Autodesk Inventor part; units mm, degrees
ref_plane "YZ Plane" through (0, 0, 0) normal (1, 0, 0) x (0, 1, 0)
ref_plane "XZ Plane" through (0, 0, 0) normal (0, 1, 0) x (-1, 0, 0)
ref_plane "XY Plane" through (0, 0, 0) normal (0, 0, 1) x (1, 0, 0)
sketch "Sketch1" plane through (0, 0, 0) normal (0, 0, 1) x (1, 0, 0)
  arc A0 (-31, -3) -> (-3, -31) centre (-3, -3) ccw
  line L0 (-31, -3) -> (-31, 0)
  line L1 (-31, 0) -> (0, 0)
  line L2 (0, 0) -> (0, -31)
  line L3 (0, -31) -> (-3, -31)
  line L4 (-31, -3) -> (-3, -3)
  line L5 (-3, -3) -> (-3, -31)
  circle A1 centre (-14.34, -15.19) radius 5.05
  circle A2 centre (-14.34, -15.19) radius 1.25
  arc A3 (0, -30.38) -> (-28.68, 0) centre (-14.34, -15.19) ccw
  dimension "wallThickness" = 3
  dimension "d1" = 3
  dimension "width" = 31
  dimension "d3" = 31
  dimension "diameter" = 10.1
  dimension "d5" = 12.19
  dimension "d6" = 11.34
  dimension "centerHoleDia" = 2.5
  dimension "setScrewRingRad" = 20.8895
extrude "Extrusion1" add sketch "Sketch1" against normal blind 3 contours L4 L5 A0 | L0 L1 L2 L3 L5 L4 | A3 L1 | L2 A3 | A1 | A2
extrude "Extrusion2" add sketch "Sketch1" along normal blind 20 contours L0 L1 L2 L3 L5 L4 | A3 L1 | L2 A3
extrude "Extrusion3" add sketch "Sketch1" along normal blind 15 contours A1 | A2
extrude "Extrusion7" cut sketch "Sketch1" along normal through all both and the other way through all contours A2
equation "\"d1\" = wallThickness"
equation "\"d3\" = width"
equation "\"d7\" = wallThickness"
properties part number "tv-mount"
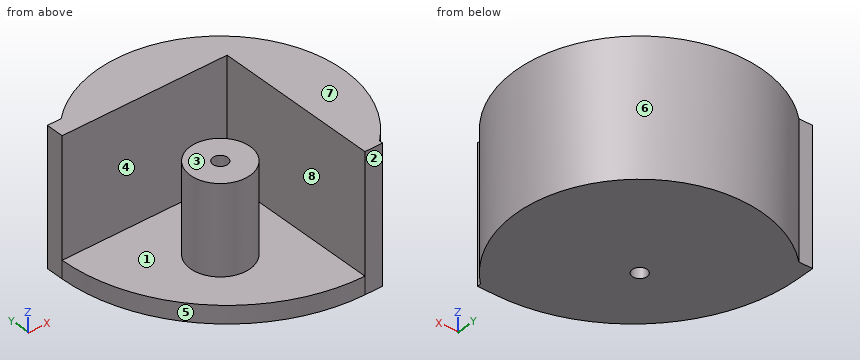
Model file for the job. Use its own axes, mm. Face numbers are marked on the shaded views. A direction names the side the tool comes from. Coordinates: 2 decimals unless noted, no trailing zeros. Order: outer loops, then holes, each group sorted by start corner. A loop starts at its lowest first (then second) coordinate and runs counter-clockwise, first axis right, second up. Notation, with made-up numbers: (37, -38) -> (80, -38) arc R7 ccw to (80, -28) -> close; hole circle Ø4 at (55, 84.5). An arc over 180 degrees is marked (long way). Answer as a JSON object with one key per item and string values. Group by question number.
1) Pull direction X, two halves, no side cores. Call the marked faces 6, 7 and 8: +X half, -X half, draft (parallel to the pull), parting line (faces both ways), or undercut.
2) Which spindle directions (+Z, -Z, +X, -X, +Y, -Y) get a long thin tool onto all of the face, cutting with end or side? Do the marked faces 1, 2, 3, 4 and 5. Say none if no direction does.
3) Cut at B-B, the plane x = -14.34. Write the cut outline in (y, z), then the cut area to 3 significant figures.
4) Drill centre lines: L1, parallel to Y at x = -14.34, z = 6.25; L2, parallel to Z at x = -20.5, y = -23; L3, parallel to Y at x = -10.5, z = 4.5. Where is each one in solid material? Low to high.
5) Flat gauge pins, fed straight in: pin 1 (3 mm diameter, centred on x = -14.34, y = -15.19, fed in from +Z); pin 2 (1.2 mm diameter, centred on x = -30, z = 7, fed in from +Y); pin 3 (1.5 mm diameter, centred on x = -22, y = -22, fed in from +Z); pin 4 (12 mm diameter, centred on x = -18.5, z = 2.5, fed in from +Y). Where does each tip first touch, or does it go through?
6) Cut at D-D, the plane y = -15.19. Write the cut outline in (x, z), then the cut area to 3 significant figures.
Check values:
{
 "1": {"face 6": "parting line", "face 7": "draft", "face 8": "undercut"},
 "2": {"face 1": "+Z", "face 2": "+Z, -Z, +X, -X, -Y", "face 3": "+Z, -X, -Y", "face 4": "+Z, -X", "face 5": "+Z, -Z, -X, -Y"},
 "3": {"outline": "(-28.6, -3) -> (-16.44, -3) -> (-16.44, 15) -> (-20.24, 15) -> (-20.24, 0) -> (-28.6, 0) -> close; (-13.94, -3) -> (5.7, -3) -> (5.7, 20) -> (-3, 20) -> (-3, 0) -> (-10.14, 0) -> (-10.14, 15) -> (-13.94, 15) -> close", "area": "383 mm²"},
 "4": {"L1": "y = -20.24 to -16.44, -13.94 to -10.14, -3 to 5.7", "L2": "z = -3 to 0", "L3": "y = -18.47 to -11.91, -3 to 5.34"},
 "5": {"pin 1": "stops at z = 15", "pin 2": "stops at y = 0", "pin 3": "stops at z = 0", "pin 4": "stops at y = 5.7"},
 "6": {"outline": "(-28.21, -3) -> (-15.59, -3) -> (-15.59, 15) -> (-19.39, 15) -> (-19.39, 0) -> (-28.21, 0) -> close; (-13.09, -3) -> (6.55, -3) -> (6.55, 20) -> (-3, 20) -> (-3, 0) -> (-9.29, 0) -> (-9.29, 15) -> (-13.09, 15) -> close", "area": "402 mm²"}
}
